```python
from build123d import *

# Parameters (mm, degrees)
SKETCH_1_R          = 5
EXTRUDE_1_DEPTH     = 5
CUT_EXTRUDE_1_DEPTH = 91.691785736
FILLET_1_R          = 2


with BuildPart() as part:
    # 草图1 → 凸台-拉伸1 (new body)
    with BuildSketch(Plane(origin=(0, 0, 0), x_dir=(1, 0, 0), z_dir=(0, 1, 0))):
        with BuildLine():
            Line((-10, 80), (-10, 0))
            ThreePointArc((-10, 0), (0, -10), (10, 0))
            Line((10, 0), (10, 80))
            ThreePointArc((10, 80), (0, 90), (-10, 80))
        make_face()
        with Locations(Location((0, 0, 0), (0, 0, 270))):
            Circle(SKETCH_1_R, mode=Mode.SUBTRACT)
        with Locations(Location((0, 80, 0), (0, 0, 270))):
            Circle(SKETCH_1_R, mode=Mode.SUBTRACT)
    extrude(amount=EXTRUDE_1_DEPTH)

    # 草图2 → 切除-拉伸1 (cut, through all)
    with BuildSketch(Plane(origin=(0, 5, 0), x_dir=(1, 0, 0), z_dir=(0, 1, 0))):
        with BuildLine():
            ThreePointArc((5, 71.339745962), (0, 70), (-5, 71.339745962))
            Line((-5, 71.339745962), (-5, 8.660254038))
            ThreePointArc((-5, 8.660254038), (0, 10), (5, 8.660254038))
            Line((5, 8.660254038), (5, 71.339745962))
        make_face()
    extrude(amount=-CUT_EXTRUDE_1_DEPTH, mode=Mode.SUBTRACT)

    # 圆角1
    fillet_1_edges = [part.edges().sort_by_distance(p)[0] for p in [
        (-5, 2.5, -71.339745962),
        (5, 2.5, -71.339745962),
        (5, 2.5, -8.660254038),
        (-5, 2.5, -8.660254038),
    ]]
    fillet(fillet_1_edges, radius=FILLET_1_R)


solid = part.part
```
Read the model definition and answer for the solid it produces. Units are mm, in the model's axes. A direction names the side the tool comes from. Give positions to 0.01 mm unless a question says otherwise; leave off trailing zeros. Write each loop counter-clockwise with the first axis right and the second up, starting at its lowest first coordinate (ties: lowest second). Pieces come first, ordered by that corner, then holes. Notation, with made-up numbers: (63.5, 71.5) - (76.5, 71.5) arc R20 ccw to (76.5, 84.5) - close; hole circle Ø3 at (17.5, 89.25). An arc over 180 degrees is marked (long way). Write item = value, one per line. Start each with the question number.
Item 1: The mould has two halves that part along Z. Classify faces 3 (the cylindrical face through (0, 2, -90)), 4 (the flat face through (-7, 0, -41)), 5 (the cylindrical face through (-4.88, 2.46, -1.08)): +Z half, -Z half, draft (parallel to the pull), parting line (faces both ways), or undercut.
Item 2: Find the intervals of material crossed by probe 1 along X at (y, z) = (2.1, -52); probe 2 along Z at (x, y) = (-1.25, 1); probe 3 along Z at (x, y) = (0.75, 1.8), in increasing order. Write a range as [from, to].
Item 3: Find section D-D (z = -78). Give the vertices of the cut face in (x, y).
Item 4: A tool of negligible diameter and unlimited length cuts with its end or side. For faces 1 (the cylindrical face through (0, 2, 10)), 2 (the cylindrical face through (0, 3, -70)), from which of +Z, -Z, +X, -X, +Y, -Y can it reach the whole face along a straight path? Write none if from no direction.
Item 5: Find section C-C (y = 3.75). Give the vertices of the cut face in (x, z), then the cut area to 3 significant figures.
Item 6: Find section A-A (x = 0). Give the vertices of the cut face in (y, z), then the cut area to 3 significant figures.
Item 7: Find section B-B (z = -25). Give the vertices of the cut face in (x, y).
Item 8: Each of these flat-tipped pins is pushed along its axis until it touches: P1, Ø3, axis at x = -3, y = 0.5, coming from the +Z side; P2, Ø8, axis at x = 0, z = -80, coming from the -Y side; P3, Ø2, axis at x = -6.5, y = 0.5, coming from the +Z side. Where does it stop, or does it pass through?
Response:
q1.face_3 = -Z half
q1.face_4 = draft
q1.face_5 = undercut
q2.probe_1 = [-10, -5], [5, 10]
q2.probe_2 = [-89.92, -84.84], [-75.16, -70.08], [-9.92, -4.84], [4.84, 9.92]
q2.probe_3 = [-89.97, -84.94], [-75.06, -70.03], [-9.97, -4.94], [4.94, 9.97]
q3.outline = (-10, 0) - (-4.58, 0) - (-4.58, 5) - (-10, 5) - close; (4.58, 0) - (10, 0) - (10, 5) - (4.58, 5) - close
q4.face_1 = +Z, +Y, -Y
q4.face_2 = +Y, -Y
q5.outline = (-10, -80) arc R10 ccw to (10, -80) - (10, 0) arc R10 ccw to (-10, 0) - close; hole circle Ø10 at (0, -80); hole (-5, -68.38) arc R2 ccw to (-2.5, -70.32) arc R10 cw to (2.5, -70.32) arc R2 ccw to (5, -68.38) - (5, -11.62) arc R2 ccw to (2.5, -9.68) arc R10 cw to (-2.5, -9.68) arc R2 ccw to (-5, -11.62) - close; hole circle Ø10 at (0, 0)
q5.area = 1,160 mm²
q6.outline = (0, -90) - (5, -90) - (5, -85) - (0, -85) - close; (0, -75) - (5, -75) - (5, -70) - (0, -70) - close; (0, -10) - (5, -10) - (5, -5) - (0, -5) - close; (0, 5) - (5, 5) - (5, 10) - (0, 10) - close
q6.area = 100 mm²
q7.outline = (-10, 0) - (-5, 0) - (-5, 5) - (-10, 5) - close; (5, 0) - (10, 0) - (10, 5) - (5, 5) - close
q8.P1 = 9.89
q8.P2 = through
q8.P3 = 8.35
